from build123d import *

# Parameters (mm, degrees)
IZIM1_W               = 300
IZIM1_H               = 150
TABAN_FLAN_1_DEPTH    = 10
IZIM2_R               = 28
KES_EKSTR_ZYON1_DEPTH = 10
IZIM3_R               = 7.5
KES_EKSTR_ZYON2_DEPTH = 10
IZIM4_R               = 7.5
KES_EKSTR_ZYON3_DEPTH = 10
IZIM5_R               = 9
KES_EKSTR_ZYON4_DEPTH = 169.002976164
IZIM8_W               = 17.5
IZIM8_H               = 33
IZIM8_W_2             = 195
SEKME1_DEPTH          = 10


# Sheet-metal steps are written as plain solids
with BuildPart() as part:
    # Çizim1 → Taban-Flanş1 (new body)
    with BuildSketch(Plane.XY):
        Rectangle(IZIM1_W, IZIM1_H)
    extrude(amount=-TABAN_FLAN_1_DEPTH)

    # Çizim2 → Kes-Ekstrüzyon1 (cut)
    with BuildSketch(Plane(origin=(0, 0, -10), x_dir=(-1, 0, 0), z_dir=(0, 0, -1))):
        with Locations((-55, -5)):
            Circle(IZIM2_R)
        with Locations((55, -5)):
            Circle(IZIM2_R)
    extrude(amount=-KES_EKSTR_ZYON1_DEPTH, mode=Mode.SUBTRACT)

    # Çizim3 → Kes-Ekstrüzyon2 (cut)
    with BuildSketch(Plane(origin=(0, 0, -10), x_dir=(-1, 0, 0), z_dir=(0, 0, -1))):
        with Locations((-137, -35)):
            Circle(IZIM3_R)
        with Locations((-137, 40)):
            Circle(IZIM3_R)
    extrude(amount=-KES_EKSTR_ZYON2_DEPTH, mode=Mode.SUBTRACT)

    # Çizim4 → Kes-Ekstrüzyon3 (cut)
    with BuildSketch(Plane(origin=(0, 0, -10), x_dir=(-1, 0, 0), z_dir=(0, 0, -1))):
        with Locations((137, -35)):
            Circle(IZIM4_R)
        with Locations((137, 40)):
            Circle(IZIM4_R)
    extrude(amount=-KES_EKSTR_ZYON3_DEPTH, mode=Mode.SUBTRACT)

    # Çizim5 → Kes-Ekstrüzyon4 (cut, through all)
    with BuildSketch(Plane(origin=(0, 0, -10), x_dir=(-1, 0, 0), z_dir=(0, 0, -1))):
        with Locations((137, -35)):
            Circle(IZIM5_R)
        with Locations((137, 40)):
            Circle(IZIM5_R)
    extrude(amount=-KES_EKSTR_ZYON4_DEPTH, mode=Mode.SUBTRACT)

    # Çizim8 → Sekme1 (add)
    with BuildSketch(Plane(origin=(0, 0, -10), x_dir=(-1, 0, 0), z_dir=(0, 0, -1))):
        with Locations((141.25, 91.5)):
            Rectangle(IZIM8_W, IZIM8_H)
        with Locations((0, 91.5)):
            Rectangle(IZIM8_W_2, IZIM8_H)
        with Locations((-141.25, 91.5)):
            Rectangle(IZIM8_W, IZIM8_H)
    extrude(amount=-SEKME1_DEPTH)


solid = part.part
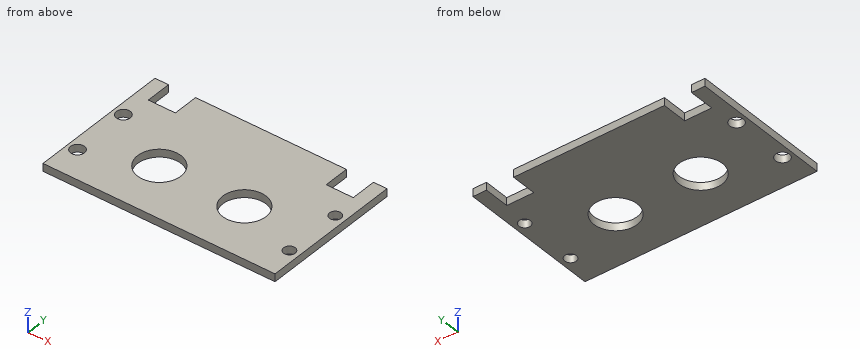
CAD build for the part. Positions are in the model's coordinates, mm. Round coordinates to 2 decimals unless told otherwise and drop trailing zeros. Loops run counter-clockwise (first coordinate to the right, second up) from the corner with the lowest first, then second, coordinate; pieces in that order, holes last.
(1) Cut at A-A (y = -5). Give the cut face in (x, z).
(2) Cut at C-C (z = -6.5). Give the cut face in (x, y), plus the area to 3 significant figures.
(3) Wall check: line 1 along Y through (x, z) = (-137, -3.75); line 2 along X through (y, z) = (77, -1.25); line 3 along Y through (x, z) = (-55, -4). Give the ranges that are in metal, low to high.
(4) Drop flat-ended pins along their axis: pin 1 (3 mm diameter, centred on x = -108, z = -4, fed in from +Y); pin 2 (11 mm diameter, centred on x = -137, y = 40, fed in from -Z). Give the stop position or say it passes through.
(5) Cut at D-D (y = 40). Give the cut face in (x, z).
(6) Cut at B-B (x = 55). Give the cut face in (y, z), plus the area to 3 significant figures.
Findings below:
1. outline: (-150, -10) - (-83, -10) - (-83, 0) - (-150, 0) - close; (-27, -10) - (27, -10) - (27, 0) - (-27, 0) - close; (83, -10) - (150, -10) - (150, 0) - (83, 0) - close
2. outline: (-150, -75) - (150, -75) - (150, 108) - (132.5, 108) - (132.5, 75) - (97.5, 75) - (97.5, 108) - (-97.5, 108) - (-97.5, 75) - (-132.5, 75) - (-132.5, 108) - (-150, 108) - close; hole circle Ø18 at (-137, -35); hole circle Ø18 at (-137, 40); hole circle Ø56 at (-55, -5); hole circle Ø56 at (55, -5); hole circle Ø15 at (137, -35); hole circle Ø15 at (137, 40)
2. area: 46,800 mm2
3. line 1: y = -75 to -44, -26 to 31, 49 to 108
3. line 2: x = -150 to -132.5, -97.5 to 97.5, 132.5 to 150
3. line 3: y = -75 to -33, 23 to 108
4. pin 1: stops at y = 75
4. pin 2: passes through
5. outline: (-150, -10) - (-146, -10) - (-146, 0) - (-150, 0) - close; (-128, -10) - (129.5, -10) - (129.5, 0) - (-128, 0) - close; (144.5, -10) - (150, -10) - (150, 0) - (144.5, 0) - close
6. outline: (-75, -10) - (-33, -10) - (-33, 0) - (-75, 0) - close; (23, -10) - (108, -10) - (108, 0) - (23, 0) - close
6. area: 1,270 mm2
